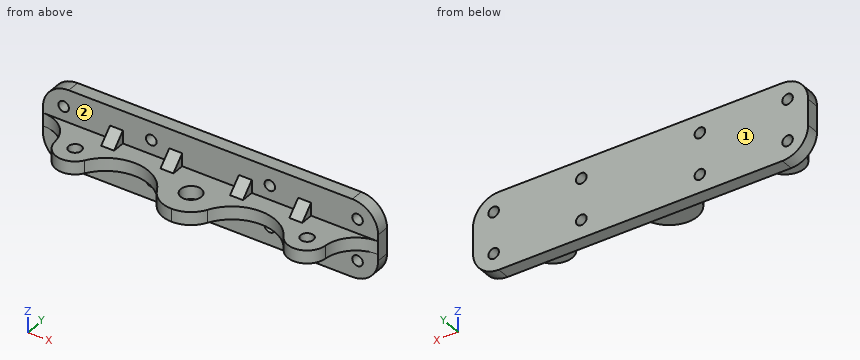
from build123d import *
from build123d.topology import SkipClean

# Parameters (mm, degrees)
SKETCH1_R                                = 2.5
BOSS_EXTRUDE1_DEPTH                      = 2.5
SKETCH4_W                                = 130
SKETCH4_H                                = 30
BOSS_EXTRUDE2_DEPTH                      = 5
FILLET1_R                                = 10
FILLET2_R                                = 12.5
SKETCH5_R                                = 2.05
CUT_EXTRUDE1_DEPTH                       = 10
BOSS_EXTRUDE3_DEPTH                      = 2.5
LPATTERN1_COUNT                          = 2
LPATTERN1_PITCH                          = 23
MIRROR4_COPY_1_DEPTH                     = 2.5
MIRROR4_AT_THE_SECOND_PLANE_COPY_1_DEPTH = 2.5
MIRROR4_AT_THE_SECOND_PLANE_COPY_2_DEPTH = 2.5
MIRROR4_AT_THE_SECOND_PLANE_COPY_3_DEPTH = 2.5


with BuildPart() as part:
    # Sketch1 → Boss-Extrude1 (new, symmetric)
    with BuildSketch(Plane.XY):
        with BuildLine():
            ThreePointArc((-38.614160498, -3.933326056), (-23.874667518, 3.933250754), (-9.779272654, -5.036449778))
            ThreePointArc((-9.779272654, -5.036449778), (-5.727087063, -9.391510729), (0, -11))
            Line((0, -11), (0, -4))
            ThreePointArc((0, -4), (-4, 0), (0, 4))
            Line((0, 4), (0, 11))
            Line((0, 11), (-52.5, 11))
            Line((-52.5, 11), (-52.5, 0))
            ThreePointArc((-52.5, 0), (-47.044040574, -7.216086067), (-38.614160498, -3.933326056))
        make_face()
        with Locations((-45, 0)):
            Circle(SKETCH1_R, mode=Mode.SUBTRACT)
    boss_extrude1 = extrude(amount=BOSS_EXTRUDE1_DEPTH, both=True)

    # Mirror1: Boss-Extrude1 across plane
    with SkipClean():  # the faces are left unmerged after this step: merging them gives an invalid solid
        add(boss_extrude1.mirror(Plane(origin=(0, 0, -2.5), x_dir=(0, 0, 1), z_dir=(-1, 0, 0))))

    # Sketch4 → Boss-Extrude2 (add)
    with SkipClean():  # the faces are left unmerged after this step: merging them gives an invalid solid
        with BuildSketch(Plane(origin=(0, 11, 0), x_dir=(1, 0, 0), z_dir=(0, 1, 0))):
            Rectangle(SKETCH4_W, SKETCH4_H)
        extrude(amount=BOSS_EXTRUDE2_DEPTH)

    # Fillet1
    fillet1_edges = [part.edges().sort_by_distance(p)[0] for p in [
        (-65, 13.5, -15),
        (-65, 13.5, 15),
        (65, 13.5, 15),
        (65, 13.5, -15),
    ]]
    fillet(fillet1_edges, radius=FILLET1_R)

    # Fillet2
    # the kernel refuses this fillet: 12.5 mm, written as the material it adds along each edge
    with BuildSketch(Plane(origin=(-52.5, 11, -2.5), x_dir=(-1, 0, 0), z_dir=(0, 0, 1))) as fillet2_piece_1:
        with BuildLine():
            CenterArc((12.443670675, 12.5), FILLET2_R, 184.301222305, 85.698777695)
            Line((-0.021123497, 11.5625), (-1.267602914, 11.46875))
            ThreePointArc((-1.267602914, 11.46875), (-1.25, 11), (-1.25, 0))
            Line((-1.25, 0), (0, -1.25))
            Line((0, -1.25), (12.443670675, -1.25))
            Line((12.443670675, -1.25), (12.443670675, 0))
        make_face()
    extrude(amount=5)
    with BuildSketch(Plane(origin=(52.5, 11, -2.5), x_dir=(1, 0, 0), z_dir=(0, 0, 1))) as fillet2_piece_2:
        with BuildLine():
            CenterArc((12.443670675, -12.5), FILLET2_R, 90, 85.698777695)
            Line((-0.021123497, -11.5625), (-1.267602914, -11.46875))
            ThreePointArc((-1.267602914, -11.46875), (-1.25, -11), (-1.25, 0))
            Line((-1.25, 0), (0, 1.25))
            Line((0, 1.25), (12.443670675, 1.25))
            Line((12.443670675, 1.25), (12.443670675, 0))
        make_face()
    extrude(amount=5)

    # Sketch5 → Cut-Extrude1 (cut)
    with BuildSketch(Plane(origin=(0, 16, 0), x_dir=(1, 0, 0), z_dir=(0, 1, 0))):
        with Locations(Location((-57, -8, 0), (0, 0, 180))):
            Circle(SKETCH5_R)
        with Locations(Location((-57, 8, 0), (0, 0, 180))):
            Circle(SKETCH5_R)
        with Locations(Location((-23, -8, 0), (0, 0, 180))):
            Circle(SKETCH5_R)
        with Locations(Location((-23, 8, 0), (0, 0, 180))):
            Circle(SKETCH5_R)
    cut_extrude1 = extrude(amount=-CUT_EXTRUDE1_DEPTH, mode=Mode.SUBTRACT)

    # Mirror2: Cut-Extrude1 across plane
    add(cut_extrude1.mirror(Plane(origin=(0, 0, 0), x_dir=(0, 0, 1), z_dir=(1, 0, 0))), mode=Mode.SUBTRACT)

    # Sketch7 → Boss-Extrude3 (add, symmetric)
    with BuildSketch(Plane(origin=(36.5, 0, 0), x_dir=(0, 0, -1), z_dir=(1, 0, 0))):
        Polygon((5, 11), (2.5, 11), (2.5, 6), (7.5, 11), align=None)
    boss_extrude3 = extrude(amount=BOSS_EXTRUDE3_DEPTH, both=True)

    # LPattern1: Boss-Extrude3 ×2
    with Locations(*[(-i * LPATTERN1_PITCH, 0, 0) for i in range(1, LPATTERN1_COUNT)]):
        add(boss_extrude3)

    # Mirror4: Boss-Extrude3 across plane
    add(boss_extrude3.mirror(Plane.XY))

    # Mirror4 copy 1 sketch → Mirror4 copy 1 (add, symmetric)
    with BuildSketch(Plane(origin=(13.5, 0, 0), x_dir=(0, 0, 1), z_dir=(1, 0, 0))):
        Polygon((5, -11), (2.5, -11), (2.5, -6), (7.5, -11), align=None)
    extrude(amount=MIRROR4_COPY_1_DEPTH, both=True)

    # Mirror4 at the second plane: Boss-Extrude3 across plane
    add(boss_extrude3.mirror(Plane(origin=(0, 0, 0), x_dir=(0, 0, 1), z_dir=(1, 0, 0))))

    # Mirror4 at the second plane copy 1 sketc → Mirror4 at the second plane copy 1 (add, symmetric)
    with BuildSketch(Plane(origin=(-13.5, 0, 0), x_dir=(0, 0, -1), z_dir=(-1, 0, 0))):
        Polygon((5, -11), (2.5, -11), (2.5, -6), (7.5, -11), align=None)
    extrude(amount=MIRROR4_AT_THE_SECOND_PLANE_COPY_1_DEPTH, both=True)

    # Mirror4 at the second plane copy 2 sketc → Mirror4 at the second plane copy 2 (add, symmetric)
    with BuildSketch(Plane.ZY.offset(36.5)):
        Polygon((5, 11), (2.5, 11), (2.5, 6), (7.5, 11), align=None)
    extrude(amount=MIRROR4_AT_THE_SECOND_PLANE_COPY_2_DEPTH, both=True)

    # Mirror4 at the second plane copy 3 sketc → Mirror4 at the second plane copy 3 (add, symmetric)
    with BuildSketch(Plane.ZY.offset(13.5)):
        Polygon((5, 11), (2.5, 11), (2.5, 6), (7.5, 11), align=None)
    extrude(amount=MIRROR4_AT_THE_SECOND_PLANE_COPY_3_DEPTH, both=True)


solid = part.part
Here's how the part is built. I have some questions about the finished solid (model axes, mm). Face numbers are marked on the shaded views. Round coordinates to 2 decimals unless told otherwise and drop trailing zeros. Write each loop counter-clockwise with the first axis right and the second up, starting at its lowest first coordinate (ties: lowest second). Pieces come first, ordered by that corner, then holes.
1. Suppose I cut it at C-C (x = 57). List the corners of the cut face in (y, z) for me.
2. Suppose I cut it at D-D (x = -6.5). List the corners of the cut face in (y, z) for me.
3. If we mould it in two halves opening along X, with no side actions, what happens to the marked faces 1 and 2? For each: released by +X, released by -X, zero draft, split by the parting line, or undercut.
4. Suppose I cut it at A-A (x = -45). List the corners of the cut face in (y, z) for me, and give its area (4 significant figures).
5. Suppose I cut it at B-B (y = 13). State how many separate pieces and enclosed holes the cut face has, and give its area (3 significant figures).
6. I need wall thicknesses on L1, parallel to Z at x = -23, y = 12.8; L2, parallel to Z at x = -57, y = 13.6; L3, parallel to X at y = -1.5, z = -0.5. Which ranges of each line are inside material? Lowest first, please.
7. Will these pins go through, and if not, where does the flat tip stop? pin 1 Ø1.5 at (y, z) = (8.5, -6) entering from -X; pin 2 Ø2 at (x, z) = (-48, 2.5) entering from -Y; pin 3 Ø2.5 at (y, z) = (8.5, 5) entering from +X.
Answer sheet:
1. outline: (8.15, -2.5) - (11, -2.5) - (11, -5.95) - (16, -5.95) - (16, 5.95) - (11, 5.95) - (11, 2.5) - (8.15, 2.5) - close; (11, -14.8) - (16, -14.8) - (16, -10.05) - (11, -10.05) - close; (11, 10.05) - (16, 10.05) - (16, 14.8) - (11, 14.8) - close
2. outline: (-8.87, -2.5) - (11, -2.5) - (11, -15) - (16, -15) - (16, 15) - (11, 15) - (11, 2.5) - (-8.87, 2.5) - close
3. face 1: zero draft
3. face 2: undercut
4. outline: (-7.5, -2.5) - (-2.5, -2.5) - (-2.5, 2.5) - (-7.5, 2.5) - close; (2.5, -2.5) - (11, -2.5) - (11, -15) - (16, -15) - (16, 15) - (11, 15) - (11, 2.5) - (2.5, 2.5) - close
4. area: 217.5 mm2
5. separate pieces: 1
5. enclosed holes: 8
5. area: 3,710 mm2
6. L1: z = -15 to -10.05, -5.95 to 5.95, 10.05 to 15
6. L2: z = -14.8 to -10.05, -5.95 to 5.95, 10.05 to 14.8
6. L3: x = -52.35 to -47, -43 to -36.79, -12.23 to -3.71, 3.71 to 12.23, 36.79 to 43, 47 to 52.35
7. pin 1: stops at x = -39
7. pin 2: stops at y = -7.23
7. pin 3: stops at x = 39
